Could you check a few things on this drawing? It's one solid part, dimensions in mm from its lowest x, y, z. A direction names the side the tool comes from. Round coordinates to 2 decimals unless told otherwise and drop trailing zeros. Loops run counter-clockwise (first coordinate to the right, second up) from the corner with the lowest first, then second, coordinate; pieces in that order, holes last. Notation, with made-up numbers: (86, -2.75) -> (90, -2.75) arc R30 cw to (90, 36.25) -> close; hole circle Ø10 at (50.5, 76). An arc over 180 degrees is marked (long way). Put each result on its own line as item: value. Start each with the question number.
1. I'm going to push flat-ended pins straight in: P1, Ø1.5, axis at y = 9, z = 57, coming from the +X side; P2, Ø1, axis at x = 17, z = 20, coming from the -Y side; P3, Ø9, axis at x = 16, y = 15.5, coming from the +Z side. Where does each tip first touch, or does it pass through?
2. Imagine slicing it at A-A, the plane x = 15. Please give me the cut outline in (y, z), and give its area (4 significant figures).
3. Imagine slicing it at D-D, the plane y = 7.5. Please give me the cut outline in (x, z), and give its area (3 significant figures).
4. Imagine slicing it at C-C, the plane z = 83.5. Please give me the cut outline in (x, y), and give its area (3 significant figures).
5. I need wall thicknesses on line 1 (Z direction, x = 9, y = 23); line 2 (Y direction, x = 15.25, z = 74.5); line 3 (Z direction, x = 24, y = 5.25). Which ranges of each line are inside material? Lowest first, please. Write a range as [from, to].
6. Imagine slicing it at B-B, the plane y = 15. Please give me the cut outline in (x, z), and give its area (3 significant figures).
7. Which directions (+Z, -Z, +X, -X, +Y, -Y) give clear straight access to the entire face, cutting with the end or side of a thin tool? Please do the marked faces 1 and 2.
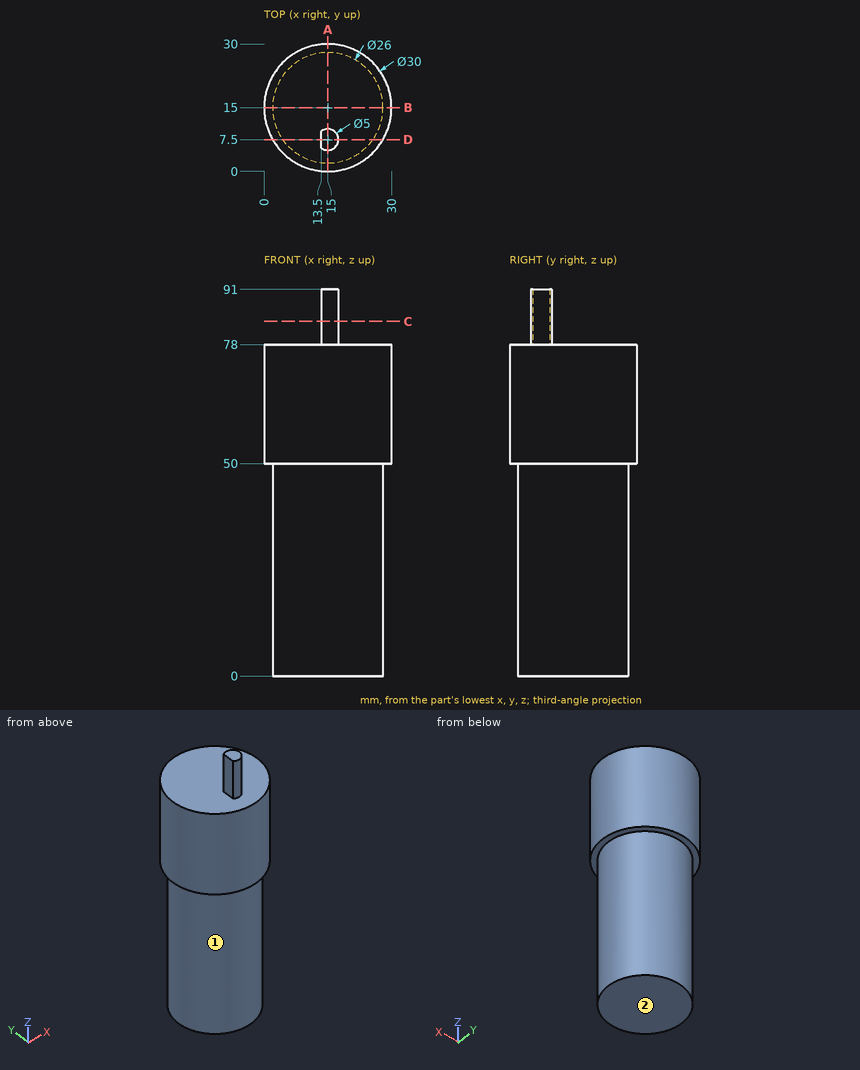
Entries:
1. P1: x = 29.05
1. P2: y = 2.09
1. P3: z = 78
2. outline: (0, 50) -> (2, 50) -> (2, 0) -> (28, 0) -> (28, 50) -> (30, 50) -> (30, 78) -> (10, 78) -> (10, 91) -> (5, 91) -> (5, 78) -> (0, 78) -> close
2. area: 2,205 mm^2
3. outline: (2.01, 50) -> (4.38, 50) -> (4.38, 0) -> (25.62, 0) -> (25.62, 50) -> (27.99, 50) -> (27.99, 78) -> (17.5, 78) -> (17.5, 91) -> (13.5, 91) -> (13.5, 78) -> (2.01, 78) -> close
3. area: 1,840 mm^2
4. outline: (13.5, 5.5) arc R2.5 ccw (long way) to (13.5, 9.5) -> close
4. area: 16.8 mm^2
5. line 1: [0, 78]
5. line 2: [0, 30]
5. line 3: [50, 78]
6. outline: (0, 50) -> (2, 50) -> (2, 0) -> (28, 0) -> (28, 50) -> (30, 50) -> (30, 78) -> (0, 78) -> close
6. area: 2,140 mm^2
7. face 1: -Z
7. face 2: -Z, +X, -X, +Y, -Y
